Geometry check sheet. Reference: the model listing, model coordinates, mm. Face numbers are marked on the shaded views. A direction names the side the tool comes from. Coordinates: 2 decimals unless noted, no trailing zeros. Loops run counter-clockwise (first coordinate to the right, second up) from the corner with the lowest first, then second, coordinate; pieces in that order, holes last. Notation, with made-up numbers: (27, 37) - (85, 37) arc R21 ccw to (85, 48) - close; hole circle Ø11 at (68.5, -32). An arc over 180 degrees is marked (long way). Write item = value, one per line. Start each with the question number.
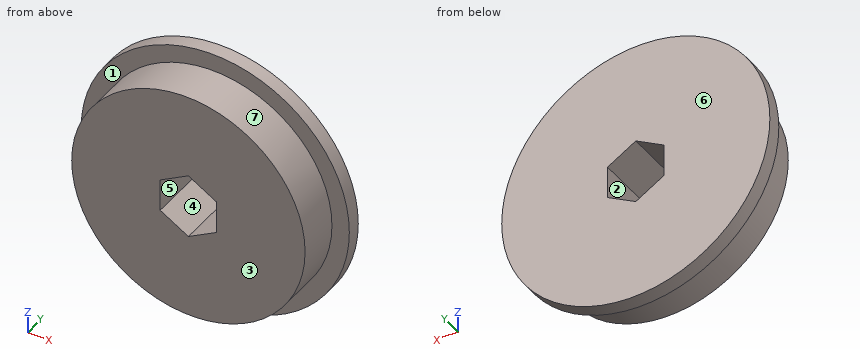
Autodesk Inventor part; units mm, degrees
ref_plane "YZ Plane" through (0, 0, 0) normal (1, 0, 0) x (0, 1, 0)
ref_plane "XZ Plane" through (0, 0, 0) normal (0, 1, 0) x (-1, 0, 0)
ref_plane "XY Plane" through (0, 0, 0) normal (0, 0, 1) x (1, 0, 0)
sketch "Sketch1" plane through (0, 0, 0) normal (0, 1, 0) x (-1, 0, 0)
  circle A0 centre (0, 0) radius 30.1625
  dimension "d0" = 60.325
extrude "Extrusion1" add sketch "Sketch1" along normal blind 3.175
sketch "Sketch2" plane through (0, 0, 0) normal (0, -1, 0) x (1, 0, 0)
  circle A0 centre (0, 0) radius 26.2509
  dimension "d3" = 52.5018
extrude "Extrusion2" add sketch "Sketch2" along normal blind 9.525
sketch "Sketch3" plane through (0, 3.175, 0) normal (0, 1, 0) x (1, 0, 0)
  line L0 (0, 7.3323) -> (6.35, 3.6662)
  line L1 (6.35, 3.6662) -> (6.35, -3.6662)
  line L2 (6.35, -3.6662) -> (0, -7.3323)
  line L3 (0, -7.3323) -> (-6.35, -3.6662)
  line L4 (-6.35, -3.6662) -> (-6.35, 3.6662)
  line L5 (-6.35, 3.6662) -> (0, 7.3323)
  point P0 (0, 0)
  point P1 (0, 0)
  dimension "d12" = 12.7
extrude "Extrusion3" cut sketch "Sketch3" against normal blind 12.7
(1) Sectioned sample at D-D on z = 24. Enter the section's corners in (x, y) (3 decimals), plus the area to 3 significant figures.
(2) Sectioned sample at B-B on y = -7. Enter the section's corners in (x, z).
(3) Sectioned sample at C-C on x = 5. Enter the section's corners in (y, z) (3 decimals).
(4) Draft check along Z on the marked faces 4, 5, 6 and 7. Enter one of: pulls with the +Z half, pulls with the -Z half, needs draft (parallel to the pull), parting line crosses it, or undercut.
(5) Depth check by flat-ended pin: pin 1 (1.5 mm diameter, centred on y = -2, z = -18.5, fed in from +X); pin 2 (5 mm diameter, centred on x = 17, y = -4.5, fed in from -Z); pin 3 (2 mm diameter, centred on y = -0.5, z = -19, fed in from -X). Enter the tip coordinate at first touch or a pass-through.
(6) Scan lines: line 1 (Y direction, x = 28.5, z = 0.5) (3 decimals); line 2 (X direction, y = -0.5, z = -1); line 3 (Z direction, x = -5.5, y = -2.75). Record each from-to range of solid material in increasing order.
(7) Tool access check on the marked faces 1, 2 and 3. Record the directions out of +Z, -Z, +X, -X, +Y, -Y that give a thin tool (end or side, any length) a straight path to the whole face; none if there is none.
Working result:
q1.outline = (-18.27, 0) - (-10.635, 0) - (-10.635, -9.525) - (10.635, -9.525) - (10.635, 0) - (18.27, 0) - (18.27, 3.175) - (-18.27, 3.175) - close
q1.area = 319 mm2
q2.outline = circle Ø52.5 at (0, 0); hole (-6.35, -3.67) - (0, -7.33) - (6.35, -3.67) - (6.35, 3.67) - (0, 7.33) - (-6.35, 3.67) - close
q3.outline = (-9.525, -25.77) - (0, -25.77) - (0, -29.745) - (3.175, -29.745) - (3.175, -4.446) - (-9.525, -4.446) - close; (-9.525, 4.446) - (3.175, 4.446) - (3.175, 29.745) - (0, 29.745) - (0, 25.77) - (-9.525, 25.77) - close
q4.face_4 = undercut
q4.face_5 = undercut
q4.face_6 = needs draft
q4.face_7 = parting line crosses it
q5.pin_1 = 19.34
q5.pin_2 = -21.88
q5.pin_3 = -24.1
q6.line_1 = 0 to 3.175
q6.line_2 = -26.23 to -6.35, 6.35 to 26.23
q6.line_3 = -25.67 to -4.16, 4.16 to 25.67
q7.face_1 = -Y
q7.face_2 = +Y, -Y
q7.face_3 = +Z, -Z, +X, -X, -Y
